```python
from build123d import *

# Parameters (mm, degrees)
EXTRUDE_1_DEPTH = 4


with BuildPart() as part:
    # 草图1 → 凸台-拉伸1 (new body)
    with BuildSketch(Plane.XY):
        Polygon((-163.090909091, -166.072727273), (-193.090909091, -134.197202987), (-193.090909091, -113.582128349), (-170.824877277, -100.726828888), (-172.824877277, -97.262727273), (-175.497524751, -98.805781011), (-175.997524751, -97.939755608), (-176.863550155, -98.439755608), (-176.363550155, -99.305781011), (-197.090909091, -111.272727273), (-197.090909091, -191.272727273), (-193.090909091, -191.272727273), (-193.090909091, -186.272727273), (-167.090909091, -186.272727273), (-167.090909091, -191.272727273), (-163.090909091, -191.272727273), align=None)
        Polygon((-193.090909091, -182.272727273), (-167.090909091, -182.272727273), (-167.090909091, -167.659017038), (-193.090909091, -140.033562656), align=None, mode=Mode.SUBTRACT)
    extrude(amount=EXTRUDE_1_DEPTH)


solid = part.part
```
Read the model definition and answer for the solid it produces. Units are mm, in the model's axes. A direction names the side the tool comes from. Give positions to 0.01 mm unless a question says otherwise; leave off trailing zeros. Write each loop counter-clockwise with the first axis right and the second up, starting at its lowest first coordinate (ties: lowest second). Pieces come first, ordered by that corner, then holes. Notation, with made-up numbers: M 3.25,73.25 L 34.25,73.25 A22 ccw 34.25,111.25 Z; hole C 89,3 d3. An arc over 180 degrees is marked long. Put each result on its own line as item: value. Start each with the question number.
1. The part is cut by section D-D, the plane y = -117.5. Give the vertices of the cut face in (x, z).
2. Which of the six approach directions +Z, -Z, +X, -X, +Y, -Y give full straight-line access (tool end or side, diameter ignored) to faces 1 (the flat face through (-180, -186.273, 2)), 2 (the flat face through (-195, -191.273, 2)), 3 (the flat face through (-182.11, -107.24, 1.97)), 4 (the flat face through (-174.1, -98, 2)), 5 (the flat face through (-179.91, -154.04, 1.97))?
3. For a pull along Y with two mould halves and no side action, classify faces 6 (the flat face through (-171.81, -99.02, 1.97)), 7 (the flat face through (-178, -154, 4)), 8 (the flat face through (-177.88, -150.36, 1.97)) as released by +Y, released by -Y, zero draft, split by the parting line, or undercut.
4. The part is cut by section B-B, the plane z = 1.55. Give the vertices of the cut face in (x, y).
5. The part is cut by section A-A, the plane y = -175. Give the vertices of the cut face in (x, z), and give its area (3 significant figures).
6. Consider line 1 along Y through (x, z) = (-176.5, 3); line 2 along Y through (x, z) = (-173, 2.85); line 3 along X through (y, z) = (-177.5, 0.75). Determine where each line is inside the solid, lowest interval first.
7. Each of these flat-tipped pins is pushed along its axis until it touches: pin 1 Ø12 at (x, y) = (-180.5, -120) entering from -Z; pin 2 Ø1.2 at (y, z) = (-160.5, 2) entering from +X; pin 3 Ø2 at (x, y) = (-190, -144.5) entering from +Z; pin 4 Ø1.2 at (x, z) = (-184, 3) entering from +Y. Where does it stop, or does it pass through?
8. The part is cut by section C-C, the plane x = -181. Give the vertices of the cut face in (y, z).
Final values:
1. outline: M -197.09,0 L -193.09,0 L -193.09,4 L -197.09,4 Z
2. face 1: +Z, -Z, -Y
2. face 2: +Z, -Z, +X, -X, -Y
2. face 3: +Z, -Z, +X
2. face 4: +Z, -Z, +Y
2. face 5: +Z, -Z
3. face 6: released by +Y
3. face 7: zero draft
3. face 8: undercut
4. outline: M -197.09,-191.27 L -193.09,-191.27 L -193.09,-186.27 L -167.09,-186.27 L -167.09,-191.27 L -163.09,-191.27 L -163.09,-166.07 L -193.09,-134.2 L -193.09,-113.58 L -170.82,-100.73 L -172.82,-97.26 L -175.5,-98.81 L -176,-97.94 L -176.86,-98.44 L -176.36,-99.31 L -197.09,-111.27 Z; hole M -193.09,-182.27 L -167.09,-182.27 L -167.09,-167.66 L -193.09,-140.03 Z
5. outline: M -197.09,0 L -193.09,0 L -193.09,4 L -197.09,4 Z; M -167.09,0 L -163.09,0 L -163.09,4 L -167.09,4 Z
5. area: 32.0 mm²
6. line 1: y = -186.27 to -182.27, -157.66 to -151.83, -104 to -99.38, -99.07 to -98.23
6. line 2: y = -186.27 to -182.27, -161.38 to -155.54, -101.98 to -97.36
6. line 3: x = -197.09 to -193.09, -167.09 to -163.09
7. pin 1: passes through
7. pin 2: stops at x = -167.77
7. pin 3: stops at z = 4
7. pin 4: stops at y = -103.37
8. outline: M -186.27,0 L -182.27,0 L -182.27,4 L -186.27,4 Z; M -152.88,0 L -147.04,0 L -147.04,4 L -152.88,4 Z; M -106.6,0 L -101.98,0 L -101.98,4 L -106.6,4 Z
